```python
from build123d import *

# Parameters (mm, degrees)
SKETCH1_R           = 82
BOSS_EXTRUDE1_DEPTH = 8
BOSS_EXTRUDE3_START = 4
BOSS_EXTRUDE3_DEPTH = 4
FILLET1_R           = 10
SKETCH8_R           = 2
CUT_EXTRUDE4_DEPTH  = 12
CIRPATTERN4_COUNT   = 3
CIRPATTERN4_ANGLE   = 180
CUT_EXTRUDE5_START  = -12
SKETCH9_R           = 1
CUT_EXTRUDE5_DEPTH  = 38
CIRPATTERN5_COUNT   = 6
CIRPATTERN5_ANGLE   = 195


with BuildPart() as part:
    # Sketch1 → Boss-Extrude1 (new body)
    with BuildSketch(Plane.XY):
        Circle(SKETCH1_R)
    extrude(amount=BOSS_EXTRUDE1_DEPTH)

    # Sketch3 → Boss-Extrude3 (add)
    with BuildSketch(Plane(origin=(0, 0, 0), x_dir=(-1, 0, 0), z_dir=(0, 0, -1)).offset(BOSS_EXTRUDE3_START)):
        with BuildLine():
            Line((10, 81.387959798), (10, 74.8348181))
            ThreePointArc((10, 74.8348181), (-75.5, 0), (10, -74.8348181))
            Line((10, -74.8348181), (10, -81.387959798))
            ThreePointArc((10, -81.387959798), (-82, 0), (10, 81.387959798))
        make_face()
    extrude(amount=-BOSS_EXTRUDE3_DEPTH)

    # Fillet1
    # the kernel refuses this fillet: 10 mm, written as the material it takes off along each edge
    with BuildSketch(Plane(origin=(-10, 74.8348181, -27.110945108), x_dir=(0, 1, 0), z_dir=(0, 0, 1))) as fillet1_piece_1:
        with BuildLine():
            CenterArc((10.660627219, -9.117486644), FILLET1_R, 114.251866349, 66.339539365)
            ThreePointArc((0.66115993, -9.22070458), (0.471837745, -4.600223565), (0, 0))
            Line((0, 0), (6.553141698, 0))
        make_face()
    extrude(amount=27.110945108, mode=Mode.SUBTRACT)
    with BuildSketch(Plane(origin=(-10, -74.8348181, -27.110945108), x_dir=(0, -1, 0), z_dir=(0, 0, 1))) as fillet1_piece_2:
        with BuildLine():
            CenterArc((10.660627219, 9.117486644), FILLET1_R, 179.408594286, 66.339539365)
            ThreePointArc((0.66115993, 9.22070458), (0.471837745, 4.600223565), (0, 0))
            Line((0, 0), (6.553141698, 0))
        make_face()
    extrude(amount=27.110945108, mode=Mode.SUBTRACT)

    # Sketch8 → Cut-Extrude4 (cut)
    with BuildSketch(Plane(origin=(0, 0, -4), x_dir=(-1, 0, 0), z_dir=(0, 0, -1))):
        with Locations((0, 82)):
            Circle(SKETCH8_R)
    cut_extrude4 = extrude(amount=-CUT_EXTRUDE4_DEPTH, mode=Mode.SUBTRACT)

    # CirPattern4: Cut-Extrude4 ×3 about axis
    cirpattern4_axis = Axis((0, 0, 0), (0, 0, -1))
    for i in range(1, CIRPATTERN4_COUNT):
        add(cut_extrude4.rotate(cirpattern4_axis, i * CIRPATTERN4_ANGLE / (CIRPATTERN4_COUNT - 1)), mode=Mode.SUBTRACT)

    # Sketch9 → Cut-Extrude5 (cut)
    with BuildSketch(Plane(origin=(0, 0, 0), x_dir=(-1, 0, 0), z_dir=(0, 0, -1)).offset(CUT_EXTRUDE5_START)):
        with Locations(Location((10, 77.356318423, 0), (0, 0, 180))):
            Circle(SKETCH9_R)
    cut_extrude5 = extrude(amount=CUT_EXTRUDE5_DEPTH, mode=Mode.SUBTRACT)

    # CirPattern5: Cut-Extrude5 ×6 about axis
    cirpattern5_axis = Axis((0, 0, 0), (0, 0, -1))
    for i in range(1, CIRPATTERN5_COUNT):
        add(cut_extrude5.rotate(cirpattern5_axis, i * CIRPATTERN5_ANGLE / (CIRPATTERN5_COUNT - 1)), mode=Mode.SUBTRACT)


solid = part.part
```
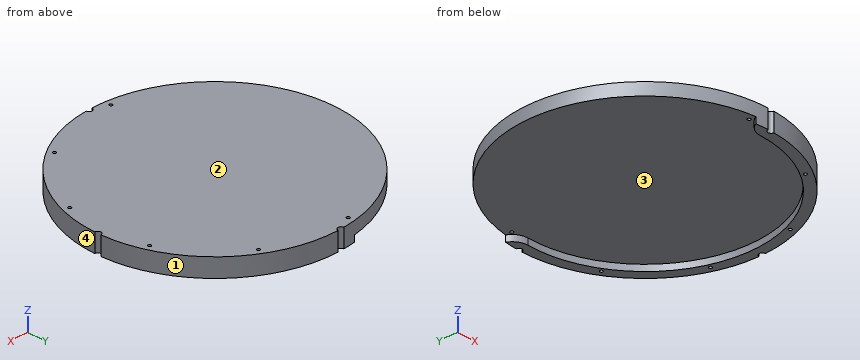
CAD build for the part. Positions are in the model's coordinates, mm. Face numbers are marked on the shaded views. Give positions to 0.01 mm unless a question says otherwise; leave off trailing zeros. Order: outer loops, then holes, each group sorted by start corner. A loop starts at its lowest first (then second) coordinate and runs counter-clockwise, first axis right, second up. Notation, with made-up numbers: M 10.5,-2 L 55.5,-2 A15 cw 55.5,18 Z; hole C 17,-29 d4. An arc over 180 degrees is marked long. Put each result on its own line as item: value. Start each with the question number.
(1) Flat gauge pins, fed straight in: pin 1 Ø2 at (y, z) = (59, -2.5) entering from -X; pin 2 Ø3 at (x, y) = (14, 48.5) entering from -Z; pin 3 Ø2 at (y, z) = (18, 2) entering from -X; pin 4 Ø1.6 at (x, y) = (-10, 77.36) entering from -Z. Where does each tip first touch, or does it go through?
(2) Saw through at A-A, the plane x = 13. Write the cut outline in (y, z), then the cut area to 3 significant figures.
(3) Mould opens along Y. For the marked faces 1, 2, 3 and 4 say: +Y half, -Y half, draft (parallel to the pull), parting line (faces both ways), or undercut.
(4) Saw through at B-B, the plane y = 0. Write the cut outline in (x, z).
(5) Drill centre lines: line 1 along Y through (x, z) = (-10, 5.75); line 2 along Y through (x, z) = (74, 3.5); line 3 along Z through (x, y) = (25, -40.5). Where is each one in solid material? Low to high.
(6) Saw through at C-C, the plane x = 32. Write the cut outline in (y, z), then the cut area to 3 significant figures.
Check result:
1. pin 1: stops at x = 45.83
1. pin 2: stops at z = 0
1. pin 3: stops at x = -80.22
1. pin 4: passes through
2. outline: M -80.96,-4 L -74.37,-4 L -74.37,0 L 74.37,0 L 74.37,-4 L 80.96,-4 L 80.96,8 L -80.96,8 Z
2. area: 1,350 mm2
3. face 1: +Y half
3. face 2: draft
3. face 3: undercut
3. face 4: -Y half
4. outline: M -82,0 L 75.5,0 L 75.5,-4 L 80,-4 L 80,8 L -82,8 Z
5. line 1: y = -81.39 to -78.24, -76.38 to 76.36, 78.36 to 81.39
5. line 2: y = -35.33 to -27.05, -25.36 to 24.95, 26.78 to 35.33
5. line 3: z = 0 to 8
6. outline: M -75.5,-4 L -68.38,-4 L -68.38,0 L 68.38,0 L 68.38,-4 L 75.5,-4 L 75.5,8 L -75.5,8 Z
6. area: 1,260 mm2
